Check sheet for the modelled part. Datum: model origin and axes. Units: mm. Round coordinates to 2 decimals unless told otherwise and drop trailing zeros. Order: outer loops, then holes, each group sorted by start corner. A loop starts at its lowest first (then second) coordinate and runs counter-clockwise, first axis right, second up.
(1) Sectioned sample at A-A, the plane x = -42.5. Enter the section's corners in (y, z), and give its area (3 significant figures).
(2) Thickness scan on probe 1 along Y at (x, z) = (42.5, 2); probe 2 along Y at (x, z) = (-41, 5.5). Record the ranges inside material, lowest first.
(3) Sectioned sample at C-C, the plane z = 2.5. Enter the section's corners in (x, y), and give its area (3 significant figures).
(4) Sectioned sample at B-B, the plane y = -25. Enter the section's corners in (x, z).
(5) Mould release check, pull along Y, two halves, no side actions. Record for faces 1 (the cylindrical face through (-45.476, -64.782, 3.169)), 2 (the flat face through (-1, -70, 3)), 3 (the flat face through (50, -1, 3)): released by +Y, released by -Y, zero draft, split by the parting line, or undercut.
```python
from build123d import *

# Parameters (mm, degrees)
F0_W     = 100
F0_H     = 140
F1_DEPTH = 6.25
F2_R     = 3.75
F3_DEPTH = 25


with BuildPart() as f1:
    # F0 (on Top) → F1 (new body)
    with BuildSketch(Plane.XY):
        Rectangle(F0_W, F0_H)
    extrude(amount=F1_DEPTH)

    # F2 (on face) → F3 (cut)
    with BuildSketch(Plane.XY.offset(6.25)):
        with Locations((-42.5, -62.5)):
            Circle(F2_R)
        with Locations((-42.5, -25)):
            Circle(F2_R)
        with Locations((-42.5, 12.5)):
            Circle(F2_R)
        with Locations((42.5, 12.5)):
            Circle(F2_R)
        with Locations((42.5, -62.5)):
            Circle(F2_R)
        with Locations((42.5, -25)):
            Circle(F2_R)
    extrude(amount=-F3_DEPTH, mode=Mode.SUBTRACT)


solid = f1.part
```
Derived:
1. outline: (-70, 0) - (-66.25, 0) - (-66.25, 6.25) - (-70, 6.25) - close; (-58.75, 0) - (-28.75, 0) - (-28.75, 6.25) - (-58.75, 6.25) - close; (-21.25, 0) - (8.75, 0) - (8.75, 6.25) - (-21.25, 6.25) - close; (16.25, 0) - (70, 0) - (70, 6.25) - (16.25, 6.25) - close
1. area: 734 mm2
2. probe 1: y = -70 to -66.25, -58.75 to -28.75, -21.25 to 8.75, 16.25 to 70
2. probe 2: y = -70 to -65.94, -59.06 to -28.44, -21.56 to 9.06, 15.94 to 70
3. outline: (-50, -70) - (50, -70) - (50, 70) - (-50, 70) - close; hole circle Ø7.5 at (-42.5, -62.5); hole circle Ø7.5 at (-42.5, -25); hole circle Ø7.5 at (-42.5, 12.5); hole circle Ø7.5 at (42.5, -62.5); hole circle Ø7.5 at (42.5, -25); hole circle Ø7.5 at (42.5, 12.5)
3. area: 13,700 mm2
4. outline: (-50, 0) - (-46.25, 0) - (-46.25, 6.25) - (-50, 6.25) - close; (-38.75, 0) - (38.75, 0) - (38.75, 6.25) - (-38.75, 6.25) - close; (46.25, 0) - (50, 0) - (50, 6.25) - (46.25, 6.25) - close
5. face 1: undercut
5. face 2: released by -Y
5. face 3: zero draft
